Verification items for the finished model (mm, model axes). A direction names the side the tool comes from. Round coordinates to 2 decimals unless told otherwise and drop trailing zeros. Write each loop counter-clockwise with the first axis right and the second up, starting at its lowest first coordinate (ties: lowest second). Pieces come first, ordered by that corner, then holes. Notation, with made-up numbers: M -19.75,26.5 L -5.75,26.5 A18 ccw -5.75,36.5 Z; hole C 27,56.25 d11. An arc over 180 degrees is marked long. One line per question, with ' | ' between items. Start each with the question number.
Q1. Release check for a two-part mould opening along Y. For faces 6 (the face through (-20, 0, 15)), 7 (the face through (0, 27, 17)), 8 (the face through (0, 32, 15)), 9 (the face through (18, -31, 15)) record: released by +Y, released by -Y, zero draft, split by the parting line, or undercut.
Q2. Cross-section at B-B (y = -9.5). Record the boundary of the cut face in (x, z).
Q3. Gauge pin test, flat ends, axial feed: pin 1 (24 mm diameter, centred on x = -2.5, y = -3, fed in from +Z); pin 2 (1.5 mm diameter, centred on x = 15, z = 56, fed in from +Y); pin 3 (6 mm diameter, centred on x = -12.5, y = 20, fed in from +Z). Record the tip position at first contact, or that the pin passes through.
Q4. Tool access check on faces 1 (the face through (-15, 0, 17)), 2 (the face through (19, 25, 58)), 3 (the face through (19, -25, 58)), 4 (the face through (0, 0, 0)), 5 (the face through (0, -32, 15)). Record the directions out of +Z, -Z, +X, -X, +Y, -Y that give a thin tool (end or side, any length) a straight path to the whole face; none if there is none.
Q5. Cross-section at A-A (z = 15). Record the boundary of the cut face in (x, y), then the cut area to 3 significant figures.
Q6. Cross-section at D-D (x = 8.5). Record the boundary of the cut face in (y, z).
Q7. Thickness scan on line 1 along Y through (x, z) = (6, 9.5); line 2 along X through (y, z) = (4.5, 29.5); line 3 along Z through (x, y) = (-9.5, -25.5). Record the ranges inside material, lowest first. Write a range as from..to.
from build123d import *

# Parameters (mm, degrees)
F0_W     = 5
F0_H     = 54
F1_DEPTH = 85
F0_W_2   = 30
F2_DEPTH = 5
F3_DEPTH = 30
F4_R     = 4.99999


# Not quite as in the source:
# - a fillet or chamfer is up to 0.001 mm smaller than in the source, because OpenCascade refuses the exact size


with BuildPart() as f1:
    # F0 (on Top) → F1 (new body)
    with BuildSketch(Plane.XY):
        with Locations((17.5, 0)):
            Rectangle(F0_W, F0_H)
    extrude(amount=F1_DEPTH)

    # F0 (on Top) → F2 (join)
    with BuildSketch(Plane.XY):
        Rectangle(F0_W_2, F0_H)
    extrude(amount=F2_DEPTH)

    # F0 (on Top) → F3 (join)
    with BuildSketch(Plane.XY):
        Polygon((20, -27), (15, -27), (-15, -27), (-15, 27), (15, 27), (20, 27), (20, 32), (-20, 32), (-20, -31.9579449729), (-20, -32), (20, -32), align=None)
    extrude(amount=F3_DEPTH)

    # F4 (radius 5 in the source; OpenCascade refuses exactly that, so slightly less here)
    f4_edges = [f1.edges().sort_by_distance(p)[0] for p in [
        (-20, -32, 15),
        (20, -32, 15),
        (20, 32, 15),
        (-20, 32, 15),
        (20, 27, 57.5),
        (20, -27, 57.5),
    ]]
    fillet(f4_edges, radius=F4_R)


solid = f1.part
Determined:
1) face 6: zero draft | face 7: undercut | face 8: released by +Y | face 9: released by -Y
2) outline: M -20,0 L 20,0 L 20,85 L 15,85 L 15,5 L -15,5 L -15,30 L -20,30 Z
3) pin 1: stops at z = 5 | pin 2: stops at y = 27 | pin 3: stops at z = 30
4) face 1: +Z | face 2: +Z, +X, +Y | face 3: +Z, +X, -Y | face 4: -Z, +X, -X, +Y, -Y | face 5: +Z, -Z, +X, -X, -Y
5) outline: M -20,-27 A5 ccw -15,-32 L 15,-32 A5 ccw 20,-27 L 20,27 A5 ccw 15,32 L -15,32 A5 ccw -20,27 Z; hole M -15,-27 L 15,-27 L 15,27 L -15,27 Z | area: 919 mm²
6) outline: M -32,0 L 32,0 L 32,30 L 27,30 L 27,5 L -27,5 L -27,30 L -32,30 Z
7) line 1: y = -32..-27, 27..32 | line 2: x = -20..-15, 15..20 | line 3: z = 0..5
